Source: CAD feature listing. Evaluate the final solid. Frame: model axes, mm. Give positions to 0.01 mm unless a question says otherwise; leave off trailing zeros. Order: outer loops, then holes, each group sorted by start corner. A loop starts at its lowest first (then second) coordinate and runs counter-clockwise, first axis right, second up. Notation, with made-up numbers: (29, -3) -> (44, -3) arc R17 cw to (44, 11) -> close; hole circle Ø9 at (12.5, 19). An arc over 180 degrees is marked (long way). Answer in a Markdown table with one row per item.
```python
from build123d import *

# Parameters (mm, degrees)
BOSS_EXTRU_1_DEPTH = 10


with BuildPart() as part:
    # Esquisse1 → Boss.-Extru.1 (new body)
    with BuildSketch(Plane(origin=(0, 0, 0), x_dir=(1, 0, 0), z_dir=(0, 1, 0))):
        with BuildLine():
            Line((-88.674901918, -25), (-88.8, -25))
            ThreePointArc((-88.8, -25), (-89.648528137, -24.648528137), (-90, -23.8))
            Line((-90, -23.8), (-90, 25))
            Line((-90, 25), (90, 25))
            Line((90, 25), (90, -23.8))
            ThreePointArc((90, -23.8), (89.648528137, -24.648528137), (88.8, -25))
            Line((88.8, -25), (88.674901918, -25))
            ThreePointArc((88.674901918, -25), (87.844302453, -24.666085752), (87.475951315, -23.850174216))
            ThreePointArc((87.475951315, -23.850174216), (60.357828362, 2.497671881), (32.56327302, -23.13559322))
            ThreePointArc((32.56327302, -23.13559322), (31.933307512, -24.461366901), (30.567874694, -25))
            Line((30.567874694, -25), (29.432125306, -25))
            ThreePointArc((29.432125306, -25), (28.066692488, -24.461366901), (27.43672698, -23.13559322))
            ThreePointArc((27.43672698, -23.13559322), (0, 2.5), (-27.43672698, -23.13559322))
            ThreePointArc((-27.43672698, -23.13559322), (-28.066692488, -24.461366901), (-29.432125306, -25))
            Line((-29.432125306, -25), (-30.567874694, -25))
            ThreePointArc((-30.567874694, -25), (-31.933307512, -24.461366901), (-32.56327302, -23.13559322))
            ThreePointArc((-32.56327302, -23.13559322), (-60.357828362, 2.497671881), (-87.475951315, -23.850174216))
            ThreePointArc((-87.475951315, -23.850174216), (-87.844302453, -24.666085752), (-88.674901918, -25))
        make_face()
    extrude(amount=BOSS_EXTRU_1_DEPTH)


solid = part.part
```
(1) Section query C-C (x = 0). Return the cut outline in (y, z), plus the area to 3 significant figures.
A:
| item | result |
|---|---|
| outline | (0, -25) -> (10, -25) -> (10, -2.5) -> (0, -2.5) -> close |
| area | 225 mm^2 |
(2) Section query B-B (y = 3). Return the cut outline in (x, z), plus the area to 3 significant figures.
A:
| item | result |
|---|---|
| outline | (-90, -25) -> (90, -25) -> (90, 23.8) arc R1.2 ccw to (88.8, 25) -> (88.67, 25) arc R1.2 ccw to (87.48, 23.85) arc R27.5 cw to (32.56, 23.14) arc R2 ccw to (30.57, 25) -> (29.43, 25) arc R2 ccw to (27.44, 23.14) arc R27.5 cw to (-27.44, 23.14) arc R2 ccw to (-29.43, 25) -> (-30.57, 25) arc R2 ccw to (-32.56, 23.14) arc R27.5 cw to (-87.48, 23.85) arc R1.2 ccw to (-88.67, 25) -> (-88.8, 25) arc R1.2 ccw to (-90, 23.8) -> close |
| area | 5,430 mm^2 |
(3) Pull-direction query (X, two-part tool) for faces 1 (the flat face through (90, 5, -1)), 2 (the flat face through (-1, 5, -25)), 3 (the cylindrical face through (-59.8, 4.9, -2.5)); classes: +X half, -X half, draft (parallel to the pull), parting line (faces both ways), or undercut.
A:
| item | result |
|---|---|
| face 1 | +X half |
| face 2 | draft |
| face 3 | undercut |
(4) Section query A-A (z = 8.5). Return the cut outline in (x, y).
A:
| item | result |
|---|---|
| outline | (-90, 0) -> (-82, 0) -> (-82, 10) -> (-90, 10) -> close; (-38, 0) -> (-22, 0) -> (-22, 10) -> (-38, 10) -> close; (22, 0) -> (38, 0) -> (38, 10) -> (22, 10) -> close; (82, 0) -> (90, 0) -> (90, 10) -> (82, 10) -> close |
(5) Ray query, probe 1 along X at (y, z) = (5.25, -0.5); probe 2 along X at (y, z) = (8, 3); probe 3 along Z at (x, y) = (60.5, 6.5). Return the intervals inside material, ascending.
A:
| item | result |
|---|---|
| probe 1 | x = -90 to -70.3, -49.7 to -10.3, 10.3 to 49.7, 70.3 to 90 |
| probe 2 | x = -90 to -76.5, -43.5 to -16.5, 16.5 to 43.5, 76.5 to 90 |
| probe 3 | z = -25 to -2.5 |
(6) Section query D-D (z = 16). Return the cut outline in (x, y), plus the area to 3 significant figures.
A:
| item | result |
|---|---|
| outline | (-90, 0) -> (-85.99, 0) -> (-85.99, 10) -> (-90, 10) -> close; (-34.01, 0) -> (-25.99, 0) -> (-25.99, 10) -> (-34.01, 10) -> close; (25.99, 0) -> (34.01, 0) -> (34.01, 10) -> (25.99, 10) -> close; (85.99, 0) -> (90, 0) -> (90, 10) -> (85.99, 10) -> close |
| area | 241 mm^2 |
(7) First-contact query: pin 1 Ø8 at (x, z) = (-22.5, 13) entering from -Y; pin 2 Ø3 at (x, y) = (-67.5, 8.5) entering from +Z; pin 3 Ø5 at (x, y) = (43, 6) entering from +Z. Flat tips, straight axial feed; report the tip coordinate or a pass-through.
A:
| item | result |
|---|---|
| pin 1 | stops at y = 0 |
| pin 2 | stops at z = -0.99 |
| pin 3 | stops at z = 5.61 |
